from build123d import *

# Parameters (mm, degrees)
ESQUISSE1_W             = 20
ESQUISSE1_H             = 42
BOSS_EXTRU_1_DEPTH      = 12
ESQUISSE2_W             = 20
ESQUISSE2_H             = 17
BOSS_EXTRU_3_DEPTH      = 14.5
ESQUISSE3_W             = 12
ESQUISSE3_H             = 12
ENL_V_MAT_EXTRU_3_DEPTH = 49.726276279
ESQUISSE4_R             = 2
ENL_V_MAT_EXTRU_4_DEPTH = 42
ENL_V_START             = -3
ENL_V_MAT_EXTRU_5_DEPTH = 6.5
ESQUISSE6_R             = 4
ENL_V_MAT_EXTRU_6_DEPTH = 13.5


with BuildPart() as part:
    # Esquisse1 → Boss.-Extru.1 (new body)
    with BuildSketch(Plane.XY):
        with Locations((10, -21)):
            Rectangle(ESQUISSE1_W, ESQUISSE1_H)
    extrude(amount=BOSS_EXTRU_1_DEPTH)

    # Esquisse2 → Boss.-Extru.3 (add)
    with BuildSketch(Plane(origin=(0, 0, 0), x_dir=(-1, 0, 0), z_dir=(0, 0, -1))):
        with Locations((-10, -33.5)):
            Rectangle(ESQUISSE2_W, ESQUISSE2_H)
    boss_extru_3 = extrude(amount=BOSS_EXTRU_3_DEPTH)

    # Esquisse3 → Enlèv. mat.-Extru.3 (cut, through all)
    with BuildSketch(Plane(origin=(20, 0, 0), x_dir=(0, 0, -1), z_dir=(1, 0, 0))):
        with Locations((6, -33.5)):
            Rectangle(ESQUISSE3_W, ESQUISSE3_H)
    enl_v_mat_extru_3 = extrude(amount=-ENL_V_MAT_EXTRU_3_DEPTH, mode=Mode.SUBTRACT)

    # Symétrie1: Boss.-Extru.3, Enlèv. mat.-Extru.3 across plane
    add(boss_extru_3.mirror(Plane(origin=(0, -21, 0), x_dir=(0, 0, 1), z_dir=(0, -1, 0))))
    add(enl_v_mat_extru_3.mirror(Plane(origin=(0, -21, 0), x_dir=(0, 0, 1), z_dir=(0, -1, 0))), mode=Mode.SUBTRACT)

    # Esquisse4 → Enlèv. mat.-Extru.4 (cut)
    with BuildSketch(Plane.XZ.offset(42)):
        with Locations(Location((13.5, -6, 0), (0, 0, 270))):
            Circle(ESQUISSE4_R)
        with Locations(Location((6.5, -6, 0), (0, 0, 270))):
            Circle(ESQUISSE4_R)
    extrude(amount=-ENL_V_MAT_EXTRU_4_DEPTH, mode=Mode.SUBTRACT)

    # Esquisse5 → Enlèv. mat.-Extru.5 (cut)
    with BuildSketch(Plane.XY.offset(12).offset(ENL_V_START)):
        Polygon((13.75277675, -27.5), (17.505553499, -21), (13.75277675, -14.5), (6.24722325, -14.5), (2.494446501, -21), (6.24722325, -27.5), align=None)
        Polygon((6.24722325, -27.5), (2.494446501, -34), (6.24722325, -40.5), (13.75277675, -40.5), (17.505553499, -34), (13.75277675, -27.5), align=None)
        Polygon((0, -40.5), (6.24722325, -40.5), (2.494446501, -34), (6.24722325, -27.5), (2.494446501, -21), (6.24722325, -14.5), (2.494446501, -8), (6.24722325, -1.5), (0, -1.5), align=None)
        Polygon((2.494446501, -8), (6.24722325, -14.5), (13.75277675, -14.5), (17.505553499, -8), (13.75277675, -1.5), (6.24722325, -1.5), align=None)
    extrude(amount=-ENL_V_MAT_EXTRU_5_DEPTH, mode=Mode.SUBTRACT)

    # Esquisse6 → Enlèv. mat.-Extru.6 (cut)
    with BuildSketch(Plane.XY.offset(12)):
        with Locations((10, -34)):
            Circle(ESQUISSE6_R)
        with Locations((10, -21)):
            Circle(ESQUISSE6_R)
        with Locations((10, -8)):
            Circle(ESQUISSE6_R)
    extrude(amount=-ENL_V_MAT_EXTRU_6_DEPTH, mode=Mode.SUBTRACT)


solid = part.part
Could you check a few things on this model? Use its own coordinates, in mm. A direction names the side the tool comes from. Coordinates: 2 decimals unless noted, no trailing zeros. Order: outer loops, then holes, each group sorted by start corner. A loop starts at its lowest first (then second) coordinate and runs counter-clockwise, first axis right, second up.
Q1. Thinking about a two-plate mould opening in X: for faces 1 (the flat face through (15.66, -30.8, 5.8)), 2 (the cylindrical face through (15.483, -15.767, -5.74)), 3 (the cylindrical face through (9.479, -30.034, 1.268)), 4 (the flat face through (4, -21, 0)), which applies, released by +X, released by -X, zero draft, split by the parting line, or undercut?
Q2. Which directions (+Z, -Z, +X, -X, +Y, -Y) give clear straight access to the entire face, cutting with the end or side of a thin tool? Please do faces 5 (the flat face through (10, 0, -1)), 6 (the flat face through (10, -34, -12)), 7 (the flat face through (15.6, -37.3, 5.8)), 8 (the flat face through (10, -25, -7)), 9 (the flat face through (10, -9, -14.5)).
Q3. Please list where these lines run through material, in increasing order: L1, parallel to Z at x = 5.5, y = -10; L2, parallel to Y at x = 10, z = 10.75; L3, parallel to Y at x = 16.5, z = -11.
Q4. Suppose I cut it at C-C on x = 17. Please give me the cut outline in (y, z).
Q5. Suppose I cut it at D-D on y = -11. Please give me the cut outline in (x, z), and give its area (3 significant figures).
Q6. Will these pins go through, and if not, where does the flat tip stop? pin 1 (5 mm diameter, centred on x = 10, y = -34, fed in from +Z); pin 2 (6.5 mm diameter, centred on x = 13.5, y = -21.5, fed in from -Z); pin 3 (1.5 mm diameter, centred on y = -23, z = 5, fed in from -X).
Q7. Suppose I cut it at B-B on z = 3.5. Please give me the cut outline in (x, y).
Q8. Suppose I cut it at A-A on y = -20.5. Please give me the cut outline in (x, z), and give its area (3 significant figures).
Answer:
1. face 1: released by -X
1. face 2: undercut
1. face 3: undercut
1. face 4: zero draft
2. face 5: +Z, -Z, +X, -X, +Y
2. face 6: +X, -X
2. face 7: -X
2. face 8: -Z, +X, -X
2. face 9: -Z, +X, -X, +Y, -Y
3. L1: z = -14.5 to -12, 0 to 2.5, 9 to 12
3. L2: y = -42 to -38, -30 to -25, -17 to -12, -4 to 0
3. L3: y = -42 to -39.5, -27.5 to -25, -17 to -14.5, -2.5 to 0
4. outline: (-42, -14.5) - (-25, -14.5) - (-25, 0) - (-17, 0) - (-17, -14.5) - (0, -14.5) - (0, 12) - (-42, 12) - close; hole (-39.5, -12) - (-27.5, -12) - (-27.5, 0) - (-39.5, 0) - close; hole (-34.88, 2.5) - (-33.12, 2.5) - (-33.12, 9) - (-34.88, 9) - close; hole (-21.88, 2.5) - (-20.12, 2.5) - (-20.12, 9) - (-21.88, 9) - close; hole (-14.5, -12) - (-2.5, -12) - (-2.5, 0) - (-14.5, 0) - close; hole (-8.88, 2.5) - (-7.12, 2.5) - (-7.12, 9) - (-8.88, 9) - close
5. outline: (0, -14.5) - (20, -14.5) - (20, -12) - (0, -12) - close; (0, 0) - (7.35, 0) - (7.35, 2.5) - (0, 2.5) - close; (0, 9) - (7.35, 9) - (7.35, 12) - (0, 12) - close; (12.65, 0) - (20, 0) - (20, 12) - (12.65, 12) - (12.65, 9) - (15.77, 9) - (15.77, 2.5) - (12.65, 2.5) - close
5. area: 158 mm2
6. pin 1: stops at z = -12
6. pin 2: stops at z = 0
6. pin 3: stops at x = 15.92
7. outline: (0, -42) - (20, -42) - (20, 0) - (0, 0) - (0, -1.5) - (13.75, -1.5) - (17.51, -8) - (13.75, -14.5) - (17.51, -21) - (13.75, -27.5) - (17.51, -34) - (13.75, -40.5) - (0, -40.5) - close
8. outline: (0, 0) - (6.03, 0) - (6.03, 2.5) - (0, 2.5) - close; (0, 9) - (6.03, 9) - (6.03, 12) - (0, 12) - close; (13.97, 0) - (20, 0) - (20, 12) - (13.97, 12) - (13.97, 9) - (17.22, 9) - (17.22, 2.5) - (13.97, 2.5) - close
8. area: 84.4 mm2
